Can you work these out from the drawing? Everything is in mm from the part's minimum corner. A direction names the side the tool comes from. Round coordinates to 2 decimals unless told otherwise and drop trailing zeros. Loops run counter-clockwise (first coordinate to the right, second up) from the corner with the lowest first, then second, coordinate; pieces in that order, holes last. Notation, with made-up numbers: (47, 58) -> (60, 58) arc R21 cw to (60, 90) -> close; hole circle Ø1 at (21.25, 46). An arc over 180 degrees is marked (long way). Use CSV: the item, a comma, the result in double quotes. Start each with the question number.
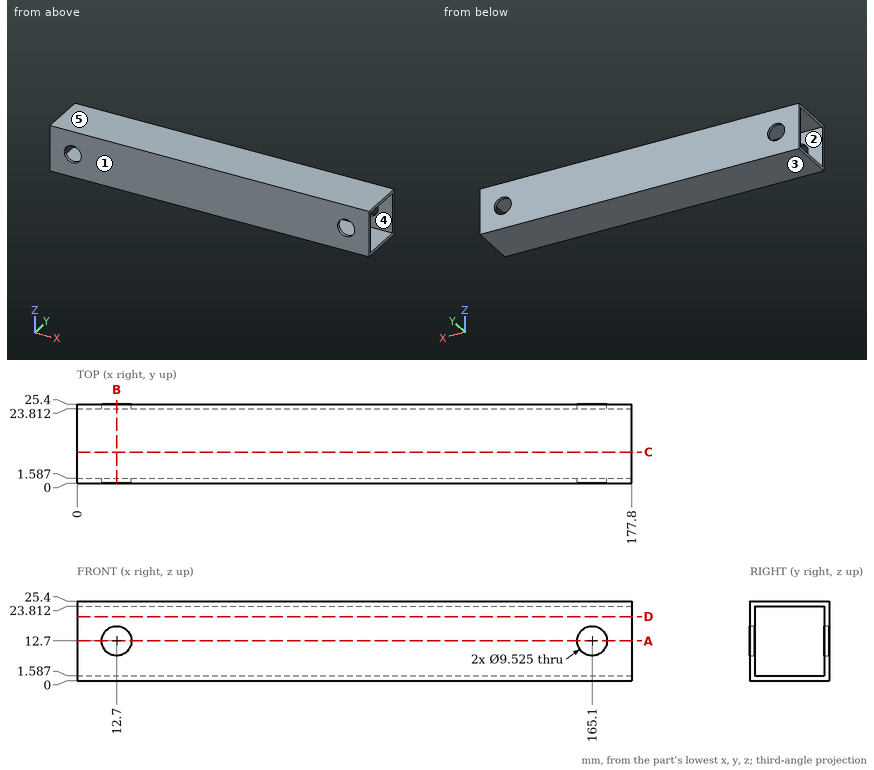
1. If I drill on L1, parallel to X at y = 0.95, z = 12.7; L2, parallel to Y at x = 44, z = 11.5, over which ranges is the centre line in solid material (lowest first)?
2. Suppose I cut it at C-C (y = 10). List the corners of the cut face in (x, z) for me.
3. Suppose I cut it at B-B (x = 12.7). List the corners of the cut face in (y, z) for me, then the cut area to 3 significant figures.
4. For the marked faces 4 and 5, which set-ups out of +Z, -Z, +X, -X, +Y, -Y let a thin tool reach every point of the face, with its end or its side?
5. Will this pin go through, and if not, where does the flat tip stop? pin 1 (2 mm diameter, centred on y = 20.5, z = 2.5, fed in from +X).
6. Suppose I cut it at A-A (z = 12.7). List the corners of the cut face in (x, y) for me.
7. We'd pull the mould along Z, two halves only. Please class the marked faces 1, 2 and 3: pulls with the +Z half, pulls with the -Z half, needs draft (parallel to the pull), parting line crosses it, or undercut.
Geometry check:
1,L1,"x = 0 to 7.94, 17.46 to 160.34, 169.86 to 177.8"
1,L2,"y = 0 to 1.59, 23.81 to 25.4"
2,outline,"(0, 0) -> (177.8, 0) -> (177.8, 1.59) -> (0, 1.59) -> close; (0, 23.81) -> (177.8, 23.81) -> (177.8, 25.4) -> (0, 25.4) -> close"
3,outline,"(0, 0) -> (25.4, 0) -> (25.4, 7.94) -> (23.81, 7.94) -> (23.81, 1.59) -> (1.59, 1.59) -> (1.59, 7.94) -> (0, 7.94) -> close; (0, 17.46) -> (1.59, 17.46) -> (1.59, 23.81) -> (23.81, 23.81) -> (23.81, 17.46) -> (25.4, 17.46) -> (25.4, 25.4) -> (0, 25.4) -> close"
3,area,"121 mm²"
4,face 4,"+X, -X"
4,face 5,"+Z, +X, -X, +Y, -Y"
5,pin 1,"stops at x = 177.8"
6,outline,"(0, 0) -> (7.94, 0) -> (7.94, 1.59) -> (0, 1.59) -> close; (0, 23.81) -> (7.94, 23.81) -> (7.94, 25.4) -> (0, 25.4) -> close; (17.46, 0) -> (160.34, 0) -> (160.34, 1.59) -> (17.46, 1.59) -> close; (17.46, 23.81) -> (160.34, 23.81) -> (160.34, 25.4) -> (17.46, 25.4) -> close; (169.86, 0) -> (177.8, 0) -> (177.8, 1.59) -> (169.86, 1.59) -> close; (169.86, 23.81) -> (177.8, 23.81) -> (177.8, 25.4) -> (169.86, 25.4) -> close"
7,face 1,"needs draft"
7,face 2,"undercut"
7,face 3,"pulls with the -Z half"
